Answer from the drawing. Dimensions are ordinates in mm from the lowest x, y and z of the part. A direction names the side the tool comes from. Give positions to 0.01 mm unless a question says otherwise; leave off trailing zeros. Order: outer loops, then holes, each group sorted by start corner. A loop starts at its lowest first (then second) coordinate and runs counter-clockwise, first axis right, second up.
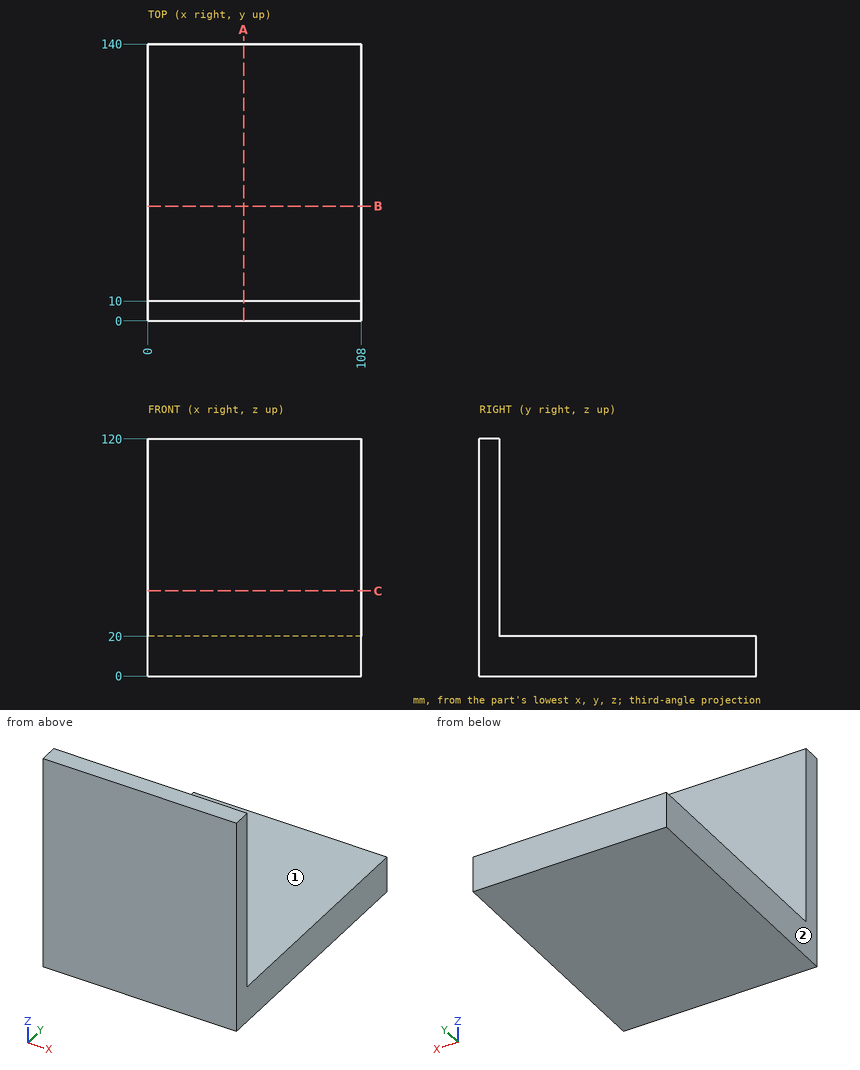
1) The part is cut by section B-B on y = 58. Determine the outline of the cut face in (x, z), and give its area (3 significant figures).
Final values:
outline: (0, 0) - (108, 0) - (108, 20) - (0, 20) - close
area: 2,160 mm2
2) Given pin 1 (1.5 mm diameter, centred on x = 53.5, y = 89.5, fed in from +Z), flat-ended and moving along its own axis, determine where the tip first touches the part or whether it passes through.
Final values:
pin 1: stops at z = 20
3) A tool of negligible diameter and unlimited length cuts with its end or side. For the marked faces 1 and 2, from which of +Z, -Z, +X, -X, +Y, -Y can it reach the whole face along a straight path? Write none if from no direction.
Final values:
face 1: +Z, +X, -X, +Y
face 2: +Z, -Z, -X, +Y, -Y
4) The part is cut by section A-A on x = 48.5. Determine the outline of the cut face in (y, z).
Final values:
outline: (0, 0) - (140, 0) - (140, 20) - (10, 20) - (10, 120) - (0, 120) - close
5) The part is cut by section C-C on z = 43. Determine the outline of the cut face in (x, y), and give its area (3 significant figures).
Final values:
outline: (0, 0) - (108, 0) - (108, 10) - (0, 10) - close
area: 1,080 mm2
6) Consider L1, parallel to Y at x = 24.5, z = 53; L2, parallel to Z at x = 22.5, y = 125. Determine where each line is inside the solid, lowest interval first.
Final values:
L1: y = 0 to 10
L2: z = 0 to 20
